Build history of the part. All positions in model axes, mm. Give positions to 0.01 mm unless a question says otherwise; leave off trailing zeros. Write each loop counter-clockwise with the first axis right and the second up, starting at its lowest first coordinate (ties: lowest second). Pieces come first, ordered by that corner, then holes. Notation, with made-up numbers: M 13,52.5 L 25,52.5 A20 cw 25,73.5 Z; hole C 40,79 d10. An arc over 180 degrees is marked long. One line per item, written item: value. Start each with the question number.
Autodesk Inventor part; units mm, degrees
ref_plane "YZ Plane" through (0, 0, 0) normal (1, 0, 0) x (0, 1, 0)
ref_plane "XZ Plane" through (0, 0, 0) normal (0, 1, 0) x (-1, 0, 0)
ref_plane "XY Plane" through (0, 0, 0) normal (0, 0, 1) x (1, 0, 0)
sketch "草圖1" plane through (0, 0, 0) normal (0, 1, 0) x (-1, 0, 0)
  line L0 (0, 0) -> (5.9088, -1.0419) construction
  line L1 (0, 0) -> (-5.9088, -1.0419) construction
  arc A0 (5.9088, -1.0419) -> (-5.9088, -1.0419) centre (0, 0) ccw
  arc A1 (-68.9365, -12.1554) -> (68.9365, -12.1554) centre (0, 0) ccw
  line L2 (5.9088, -1.0419) -> (68.9365, -12.1554)
  line L3 (-5.9088, -1.0419) -> (-68.9365, -12.1554)
  circle A2 centre (23.5124, -38.3688) radius 22.5
  circle A3 centre (-23.5124, -38.3688) radius 22.5 construction
  arc A4 (-23.5124, -38.3688) -> (23.5124, -38.3688) centre (0, 0) ccw construction
  line L4 (23.5124, -38.3688) -> (0, 0) construction
  line L5 (-23.5124, -38.3688) -> (0, 0) construction
  line L6 (0, -85.2185) -> (0, 21.3111) construction
  line L7 (69.7247, -6.2018) -> (0, 6.0926)
  line L8 (0, 6.0926) -> (-69.7247, -6.2018)
  arc A5 (68.9365, -12.1554) -> (69.7247, -6.2018) centre (0, 0) ccw
  arc A6 (-69.7247, -6.2018) -> (-68.9365, -12.1554) centre (0, 0) ccw
  dimension "d0" = 12
  dimension "d1" = 45
  dimension "d3" = 45
  dimension "d5" = 160
  dimension "d6" = 63
  dimension "d7" = 70
extrude "擠出1" add sketch "草圖1" against normal blind 2
hole "孔1" at (0, 0, 0) direction (0, -1, 0) diameter 3.2 end through all
sketch "草圖2" plane through (0, 0, 0) normal (0, 1, 0) x (-1, 0, 0)
  arc A0 (-23.5124, -38.3688) -> (23.5124, -38.3688) centre (0, 0) ccw construction
  circle A1 centre (0, 0) radius 1.6
  circle A2 centre (0, 0) radius 45
feature "擠出表面1" [suppressed]
sketch "草圖3" plane through (0, -2, 0) normal (0, -1, 0) x (1, 0, 0)
  circle A0 centre (0, -13.25) radius 0.75
  circle A1 centre (0, -16.25) radius 0.75
  circle A2 centre (0, -10.25) radius 0.75
  circle A3 centre (0, -7.25) radius 0.75
  line L0 (0, 0) -> (0, -16.25) construction
  circle A4 centre (0, 0) radius 1.6 construction
  circle A5 centre (13.25, 0) radius 0.75
  circle A6 centre (16.25, 0) radius 0.75
  circle A7 centre (10.25, 0) radius 0.75
  circle A8 centre (7.25, 0) radius 0.75
  circle A9 centre (0, 13.25) radius 0.75
  circle A10 centre (0, 16.25) radius 0.75
  circle A11 centre (0, 10.25) radius 0.75
  circle A12 centre (0, 7.25) radius 0.75
  circle A13 centre (-13.25, 0) radius 0.75
  circle A14 centre (-16.25, 0) radius 0.75
  circle A15 centre (-10.25, 0) radius 0.75
  circle A16 centre (-7.25, 0) radius 0.75
  dimension "d21" = 3
  dimension "d22" = 3
  dimension "d24" = 1.5
  dimension "d25" = 3
  dimension "d26" = 7.25
  dimension "d29" = 360
hole "孔2" at (-7.25, -2, 0) at (-10.25, -2, 0) at (-13.25, -2, 0) at (-16.25, -2, 0) at (0, -2, -13.25) at (0, -2, -16.25) at (0, -2, -7.25) at (0, -2, -10.25) at (7.25, -2, 0) at (10.25, -2, 0) at (13.25, -2, 0) at (16.25, -2, 0) direction (0, 1, 0) diameter 2 end through all
properties part number "A0002"
1) Probe line 1 along Z through (x, y) = (-10.25, -0.7); line 2 along Z through (x, y) = (0, -0.7); line 3 along Z through (x, y) = (-16.25, -0.8). List the from-to ranges inside material, lowest first. Write a range as from..to.
2) Drop flat-ended pins along their axis: P1, Ø2.5, axis at x = 0, z = -7.25, coming from the -Y side; P2, Ø1.6, axis at x = -7.25, z = 0, coming from the -Y side. Give the stop position or say it passes through.
3) Band-saw the part on A-A (y = -1.7). Count the separate pieces of the cut face and the enclosed holes in it, then the cut area to 3 significant figures.
4) Band-saw the part on B-B (z = -26). List the corners of the cut face in (x, y), then the cut area to 3 significant figures.
5) Band-saw the part on C-C (x = 31). List the corners of the cut face in (y, z), then the cut area to 3 significant figures.
6) Band-saw the part on D-D (z = -44). List the corners of the cut face in (x, y), then the cut area to 3 significant figures.
7) Mould opens along Z. For faces 1 (the face through (1, -2, -23)), 2 (the face through (-35.35, -0.99, -0.14)), 3 (the face through (0.97, -1.01, -1.27)) say: released by +Z, released by -Z, zero draft, split by the parting line, or undercut.
Model answer:
1. line 1: z = -69.25..-56.54, -20.19..-1, 1..4.29
1. line 2: z = -70..-17.25, -15.25..-14.25, -12.25..-11.25, -9.25..-8.25, -6.25..-1.6, 1.6..6.09
1. line 3: z = -68.09..-59.66, -17.07..-1, 1..3.23
2. P1: stops at y = -2
2. P2: passes through
3. separate pieces: 1
3. enclosed holes: 14
3. area: 6,050 mm²
4. outline: M -64.99,-2 L -42.31,-2 L -42.31,0 L -64.99,0 Z; M -4.72,-2 L 64.99,-2 L 64.99,0 L -4.72,0 Z
4. area: 185 mm²
5. outline: M -2,-62.76 L 0,-62.76 L 0,0.63 L -2,0.63 Z
5. area: 127 mm²
6. outline: M -54.44,-2 L -45.3,-2 L -45.3,0 L -54.44,0 Z; M -1.73,-2 L 54.44,-2 L 54.44,0 L -1.73,0 Z
6. area: 131 mm²
7. face 1: zero draft
7. face 2: released by +Z
7. face 3: undercut
